Build history of the part. All positions in model axes, mm. A direction names the side the tool comes from. Round coordinates to 2 decimals unless told otherwise and drop trailing zeros. Loops run counter-clockwise (first coordinate to the right, second up) from the corner with the lowest first, then second, coordinate; pieces in that order, holes last.
from build123d import *

# Parameters (mm, degrees)
F0_R     = 2.5
F1_DEPTH = 10


with BuildPart() as f1:
    # F0 (on Top) → F1 (new body)
    with BuildSketch(Plane.XY):
        with BuildLine():
            ThreePointArc((10.269494, -4.949495), (11.11378, -2.538481), (11.4, 0))
            ThreePointArc((11.4, 0), (11.11378, 2.538481), (10.269494, 4.949495))
            Line((10.269494, 4.949495), (4.95, 4.949495))
            Line((4.95, 4.949495), (4.95, 10.26925))
            ThreePointArc((4.95, 10.26925), (0, 11.4), (-4.95, 10.26925))
            Line((-4.95, 10.26925), (-4.95, 4.949495))
            Line((-4.95, 4.949495), (-10.269494, 4.949495))
            ThreePointArc((-10.269494, 4.949495), (-11.4, 0), (-10.269494, -4.949495))
            Line((-10.269494, -4.949495), (-4.95, -4.949495))
            Line((-4.95, -4.949495), (-4.95, -10.26925))
            ThreePointArc((-4.95, -10.26925), (0, -11.4), (4.95, -10.26925))
            Line((4.95, -10.26925), (4.95, -4.949495))
            Line((4.95, -4.949495), (10.269494, -4.949495))
        make_face()
        with Locations((0, -7)):
            Circle(F0_R, mode=Mode.SUBTRACT)
        Circle(F0_R, mode=Mode.SUBTRACT)
    extrude(amount=F1_DEPTH)


solid = f1.part
(1) Which spindle directions (+Z, -Z, +X, -X, +Y, -Y) get a long thin tool onto all of the face, cutting with end or side? Do faces 1 (the face through (4.95, 8, 5)), 2 (the face through (-8, -4.949, 5)), 3 (the face through (-0.54, -9.44, 4.93)), 4 (the face through (-8, 4.949, 5)), 5 (the face through (4.95, -8, 5)). Say none if no direction does.
Responses:
face 1: +Z, -Z, +X, +Y
face 2: +Z, -Z, -X, -Y
face 3: +Z, -Z
face 4: +Z, -Z, -X, +Y
face 5: +Z, -Z, +X, -Y
(2) Pull direction X, two halves, no side cores. Call faces 6 (the face through (8, -4.949, 5)), 7 (the face through (-11.4, 0.1, 4.9)), 8 (the face through (-0.54, -2.44, 4.93)): +X half, -X half, draft (parallel to the pull), parting line (faces both ways), or undercut.
Responses:
face 6: draft
face 7: -X half
face 8: undercut
(3) Slice it at C-C on z = 5. List the corners of the cut face in (x, y).
Responses:
outline: (-10.27, -4.95) - (-4.95, -4.95) - (-4.95, -10.27) arc R11.4 ccw to (4.95, -10.27) - (4.95, -4.95) - (10.27, -4.95) arc R11.4 ccw to (11.4, 0) arc R11.4 ccw to (10.27, 4.95) - (4.95, 4.95) - (4.95, 10.27) arc R11.4 ccw to (-4.95, 10.27) - (-4.95, 4.95) - (-10.27, 4.95) arc R11.4 ccw to start; hole circle Ø5 at (0, -7); hole circle Ø5 at (0, 0)
(4) Slice it at D-D on y = 9.5. List the corners of the cut face in (x, z), plus the area to 3 significant figures.
Responses:
outline: (-4.95, 0) - (4.95, 0) - (4.95, 10) - (-4.95, 10) - close
area: 99.0 mm2
(5) Pin check, flat tips, straight feed: P1, Ø1.6, axis at y = 6.5, z = 7, coming from the +X side; P2, Ø4, axis at y = -6, z = 4, coming from the -X side; P3, Ø3, axis at x = -5, z = 5.5, coming from the -Y side; P4, Ø1, axis at x = -0.5, y = -1, coming from the +Z side. Stop position of each tip, or through.
Responses:
P1: stops at x = 4.95
P2: stops at x = -10.68
P3: stops at y = -10.85
P4: passes through
(6) Probe line 1 (Y direction, x = 0, z = 4); line 2 (Y direction, x = 1, z = 7.5); line 3 (Y direction, x = 6.25, z = 5.5). List the from-to ranges inside material, lowest first.
Responses:
line 1: y = -11.4 to -9.5, -4.5 to -2.5, 2.5 to 11.4
line 2: y = -11.36 to -9.29, -4.71 to -2.29, 2.29 to 11.36
line 3: y = -4.95 to 4.95
(7) Slice it at A-A on y = -5.5. List the corners of the cut face in (x, z), plus the area to 3 significant figures.
Responses:
outline: (-4.95, 0) - (-2, 0) - (-2, 10) - (-4.95, 10) - close; (2, 0) - (4.95, 0) - (4.95, 10) - (2, 10) - close
area: 59.0 mm2
(8) Slice it at B-B on x = 0. List the corners of the cut face in (y, z), plus the area to 3 significant figures.
Responses:
outline: (-11.4, 0) - (-9.5, 0) - (-9.5, 10) - (-11.4, 10) - close; (-4.5, 0) - (-2.5, 0) - (-2.5, 10) - (-4.5, 10) - close; (2.5, 0) - (11.4, 0) - (11.4, 10) - (2.5, 10) - close
area: 128 mm2
